Source: CAD feature listing. Evaluate the final solid. Frame: model axes, mm. A direction names the side the tool comes from. Give positions to 0.01 mm unless a question says otherwise; leave off trailing zeros. Loops run counter-clockwise (first coordinate to the right, second up) from the corner with the lowest first, then second, coordinate; pieces in that order, holes last.
```python
from build123d import *

# Parameters (mm, degrees)
F0_W      = 115.5085265636
F0_H      = 107.8471690416
F0_W_2    = 17.5325423479
F0_H_2    = 23.7205028534
F1_DEPTH  = 127
F2_R      = 55.6100218135
F2_R_2    = 41.4969022391
F2_R_3    = 27.3255706414
F2_R_4    = 11.4895056952
F2_R_5    = 7.610471178
F3_DEPTH  = 25.4
F4_W      = 64.0326142311
F4_H      = 62.4924302101
F4_W_2    = 30.7222977281
F4_H_2    = 33.4180146456
F5_DEPTH  = 25.4
F6_W      = 61.6823285818
F6_H      = 65.940104425
F6_W_2    = 35.1780280471
F6_H_2    = 32.1564599872
F7_DEPTH  = 25.4
F8_W      = 82.6514363289
F8_H      = 73.6512206495
F8_W_2    = 46.7445999384
F8_H_2    = 39.9785265326
F9_DEPTH  = 25.4
F10_W     = 81.0015127063
F10_H     = 71.895327419
F10_W_2   = 39.0375070274
F10_H_2   = 38.2135286927
F11_DEPTH = 25.4
F12_R     = 48.8134428036
F12_R_2   = 30.6319229548
F12_R_3   = 9.5593039908
F13_DEPTH = 25.4


with BuildPart() as f1:
    # F0 (on Top) → F1 (new body)
    with BuildSketch(Plane.XY):
        Rectangle(F0_W, F0_H)
        with Locations((-66.5205344558, 0)):
            Rectangle(F0_W_2, F0_H)
        with Locations((0, 65.7838359475)):
            Rectangle(F0_W, F0_H_2)
        with Locations((66.5205344558, 0)):
            Rectangle(F0_W_2, F0_H)
        with Locations((0, -65.7838359475)):
            Rectangle(F0_W, F0_H_2)
    extrude(amount=F1_DEPTH)

    # F2 (on face) → F3 (join)
    with BuildSketch(Plane.XY.offset(127)):
        Circle(F2_R)
        Circle(F2_R_2, mode=Mode.SUBTRACT)
        Circle(F2_R_2)
        Circle(F2_R_3, mode=Mode.SUBTRACT)
        Circle(F2_R_4)
        Circle(F2_R_5, mode=Mode.SUBTRACT)
    extrude(amount=F3_DEPTH)

    # F4 (on face) → F5 (join)
    with BuildSketch(Plane.YZ.offset(75.2868056297)):
        with Locations((0, 68.5164183378)):
            Rectangle(F4_W, F4_H)
        with Locations((0, 68.5164183378)):
            Rectangle(F4_W_2, F4_H_2, mode=Mode.SUBTRACT)
    extrude(amount=F5_DEPTH)

    # F6 (on face) → F7 (join)
    with BuildSketch(Plane(origin=(0, 77.6440873742, 0), x_dir=(-1, 0, 0), z_dir=(0, 1, 0))):
        with Locations((0, 61.1903108656)):
            Rectangle(F6_W, F6_H)
        with Locations((0, 61.1903108656)):
            Rectangle(F6_W_2, F6_H_2, mode=Mode.SUBTRACT)
    extrude(amount=F7_DEPTH)

    # F8 (on face) → F9 (join)
    with BuildSketch(Plane.XZ.offset(77.6440873742)):
        with Locations((0, 64.0937909484)):
            Rectangle(F8_W, F8_H)
        with Locations((0, 64.0937909484)):
            Rectangle(F8_W_2, F8_H_2, mode=Mode.SUBTRACT)
    extrude(amount=F9_DEPTH)

    # F10 (on face) → F11 (join)
    with BuildSketch(Plane(origin=(-75.2868056297, 0, 0), x_dir=(0, -1, 0), z_dir=(-1, 0, 0))):
        with Locations((0, 66.6888132691)):
            Rectangle(F10_W, F10_H)
        with Locations((0, 66.6888132691)):
            Rectangle(F10_W_2, F10_H_2, mode=Mode.SUBTRACT)
    extrude(amount=F11_DEPTH)

    # F12 (on face) → F13 (join)
    with BuildSketch(Plane(origin=(0, 0, 0), x_dir=(1, 0, 0), z_dir=(0, 0, -1))):
        Circle(F12_R)
        Circle(F12_R_2, mode=Mode.SUBTRACT)
        Circle(F12_R_3)
    extrude(amount=F13_DEPTH)


solid = f1.part
```
(1) Section B-B, the plane y = 88.5. Return the cut outline in (x, z), then the cut area to 3 significant figures.
A:
outline: (-30.84, 28.22) - (30.84, 28.22) - (30.84, 94.16) - (-30.84, 94.16) - close; hole (-17.59, 45.11) - (17.59, 45.11) - (17.59, 77.27) - (-17.59, 77.27) - close
area: 2,940 mm2
(2) Section C-C, the plane y = 45. Return the cut outline in (x, z), then the cut area to 3 significant figures.
A:
outline: (-75.29, 0) - (-18.91, 0) - (-18.91, -25.4) - (18.91, -25.4) - (18.91, 0) - (75.29, 0) - (75.29, 127) - (32.67, 127) - (32.67, 152.4) - (-32.67, 152.4) - (-32.67, 127) - (-75.29, 127) - close
area: 21,700 mm2
(3) Section A-A, the plane z = -6.5. Return the cut outline in (x, y).
A:
outline: circle Ø97.63 at (0, 0); circle Ø19.12 at (0, 0); hole circle Ø61.26 at (0, 0)
(4) Mould query, pull axis X, two halves, no side actions, for faces 1 (the flat face through (17.589, 90, 61)), 2 (the flat face through (30.841, 90, 61)), 3 (the flat face through (-20, 103.044, 62)). Classes: pulls with the +X half, pulls with the -X half, needs draft (parallel to the pull), parting line crosses it, or undercut.
A:
face 1: undercut
face 2: pulls with the +X half
face 3: needs draft
(5) Section D-D, the plane x = -72. Return the cut outline in (y, z), then the cut area to 3 significant figures.
A:
outline: (-53.92, 0) - (53.92, 0) - (53.92, 127) - (-53.92, 127) - close
area: 13,700 mm2
(6) Ray query, line 1 along Y through (x, z) = (0, 135); line 2 along X through (y, z) = (0, -9). Return the intervals inside material, ascending.
A:
line 1: y = -55.61 to -27.33, -11.49 to -7.61, 7.61 to 11.49, 27.33 to 55.61
line 2: x = -48.81 to -30.63, -9.56 to 9.56, 30.63 to 48.81
(7) First-contact query: pin 1 (20.5 mm diameter, centred on x = 89.5, y = -10.5, fed in from -Z); pin 2 (10 mm diameter, centred on y = 66, z = 1, fed in from +X); pin 3 (19.5 mm diameter, centred on x = 68, z = 67, fed in from +Y). Flat tips, straight axial feed; report the tip coordinate or a pass-through.
A:
pin 1: stops at z = 37.27
pin 2: stops at x = 57.75
pin 3: stops at y = 53.92
(8) Reachability of faces 4 (the flat face through (-88, -40.501, 66)), 5 (the flat face through (0, -90, 84.083)), 6 (the flat face through (0, 0, 127)), 7 (the flat face through (-88, 19.519, 66)), 8 (the flat face through (-35, 36, 0)) from +Z, -Z, +X, -X, +Y, -Y: full face, straight path, thin tool, end or side. Return the list, or none.
A:
face 4: +Z, -Z, -X, -Y
face 5: -Y
face 6: +Z
face 7: -X
face 8: -Z
